```python
from build123d import *

# Parameters (mm, degrees)
F2_R     = 3.1877
F3_DEPTH = 25.4


with BuildPart() as f1:
    # F0 (on Front) → F1 (revolve)
    with BuildSketch(Plane.XZ):
        Polygon((11.1125, 50.8), (11.1125, 0), (28.575, 0), (28.575, 4.7625), (15.875, 4.7625), (15.875, 50.8), align=None)
    revolve(axis=Axis((0, 0, 24.967514), (0, 0, 1)))

    # F2 (on face) → F3 (cut)
    with BuildSketch(Plane.XY.offset(4.7625)):
        with Locations((0, 22.225)):
            Circle(F2_R)
        with Locations((19.247415, 11.1125)):
            Circle(F2_R)
        with Locations((19.247415, -11.1125)):
            Circle(F2_R)
        with Locations((0, -22.225)):
            Circle(F2_R)
        with Locations((-19.247415, -11.1125)):
            Circle(F2_R)
        with Locations((-19.247415, 11.1125)):
            Circle(F2_R)
    extrude(amount=-F3_DEPTH, mode=Mode.SUBTRACT)


solid = f1.part
```
Could you check a few things on this model? Use its own coordinates, in mm. A direction names the side the tool comes from. Round coordinates to 2 decimals unless told otherwise and drop trailing zeros. Loops run counter-clockwise (first coordinate to the right, second up) from the corner with the lowest first, then second, coordinate; pieces in that order, holes last. Notation, with made-up numbers: M 12,-30.75 L 71,-30.75 A23 cw 71,-18.75 Z; hole C 8,50 d6. An arc over 180 degrees is marked long. Write item = value, one per line.
1. I need wall thicknesses on probe 1 along Y at (x, z) = (0, 2.7) (1 decimal); probe 2 along X at (y, z) = (-0.5, 31). Which ranges of each line are inside material? Lowest first, please.
Results below:
probe_1 = -28.6 to -25.4, -19 to -11.1, 11.1 to 19, 25.4 to 28.6
probe_2 = -15.87 to -11.1, 11.1 to 15.87
2. I want a section at A-A, the plane x = 0. Write out the boundary of the cut face in (y, z) (1 decimal), and give its area (3 significant figures).
Results below:
outline = M -28.6,0 L -25.4,0 L -25.4,4.8 L -28.6,4.8 Z; M -19,0 L -11.1,0 L -11.1,50.8 L -15.9,50.8 L -15.9,4.8 L -19,4.8 Z; M 11.1,0 L 19,0 L 19,4.8 L 15.9,4.8 L 15.9,50.8 L 11.1,50.8 Z; M 25.4,0 L 28.6,0 L 28.6,4.8 L 25.4,4.8 Z
area = 544 mm²
3. I want a section at B-B, the plane y = 0. Write out the boundary of the cut face in (x, z) (1 decimal).
Results below:
outline = M -28.6,0 L -11.1,0 L -11.1,50.8 L -15.9,50.8 L -15.9,4.8 L -28.6,4.8 Z; M 11.1,0 L 28.6,0 L 28.6,4.8 L 15.9,4.8 L 15.9,50.8 L 11.1,50.8 Z
4. I want a section at C-C, the plane x = -9.5. Write out the boundary of the cut face in (y, z).
Results below:
outline = M -26.95,0 L -5.77,0 L -5.77,50.8 L -12.72,50.8 L -12.72,4.76 L -26.95,4.76 Z; M 5.77,0 L 26.95,0 L 26.95,4.76 L 12.72,4.76 L 12.72,50.8 L 5.77,50.8 Z
5. Will these pins go through, and if not, where does the flat tip stop? P1, Ø10, axis at y = 12, z = 27, coming from the -X side; P2, Ø8.5, axis at x = 19.25, y = 11.11, coming from the +Z side; P3, Ø8, axis at y = -1.5, z = 10.5, coming from the -X side (3 decimals); P4, Ø5, axis at x = 0, y = -22.225, coming from the -Z side.
Results below:
P1 = -14.25
P2 = 4.76
P3 = -15.875
P4 = through
6. Thinking about a two-plate mould opening in Y: for faces 3 (the face through (-12, 0, 0)), 4 (the face through (-3.441, -15.497, 28.104)), 5 (the face through (-0.691, -25.337, 2.415)), 6 (the face through (-0.415, 25.386, 2.415)), which applies, +Y half, -Y half, draft (parallel to the pull), parting line (faces both ways), or undercut?
Results below:
face_3 = draft
face_4 = parting line
face_5 = undercut
face_6 = undercut
7. Which directions (+Z, -Z, +X, -X, +Y, -Y) give clear straight access to the entire face, cutting with the end or side of a thin tool? Please do faces 1 (the face through (12, -12, 4.762)), 2 (the face through (-28.547, 1.256, 2.415)).
Results below:
face_1 = +Z
face_2 = +Z, -Z
